Print and shaded views of the part. All mm, measured from the part's lowest x, y and z. A direction names the side the tool comes from. Round coordinates to 2 decimals unless told otherwise and drop trailing zeros. Loops run counter-clockwise (first coordinate to the right, second up) from the corner with the lowest first, then second, coordinate; pieces in that order, holes last. Notation, with made-up numbers: M 34,24.5 L 63,24.5 A9 ccw 63,30.5 Z; hole C -24.75,12.5 d9. An arc over 180 degrees is marked long. One line per item, written item: value. Start each with the question number.
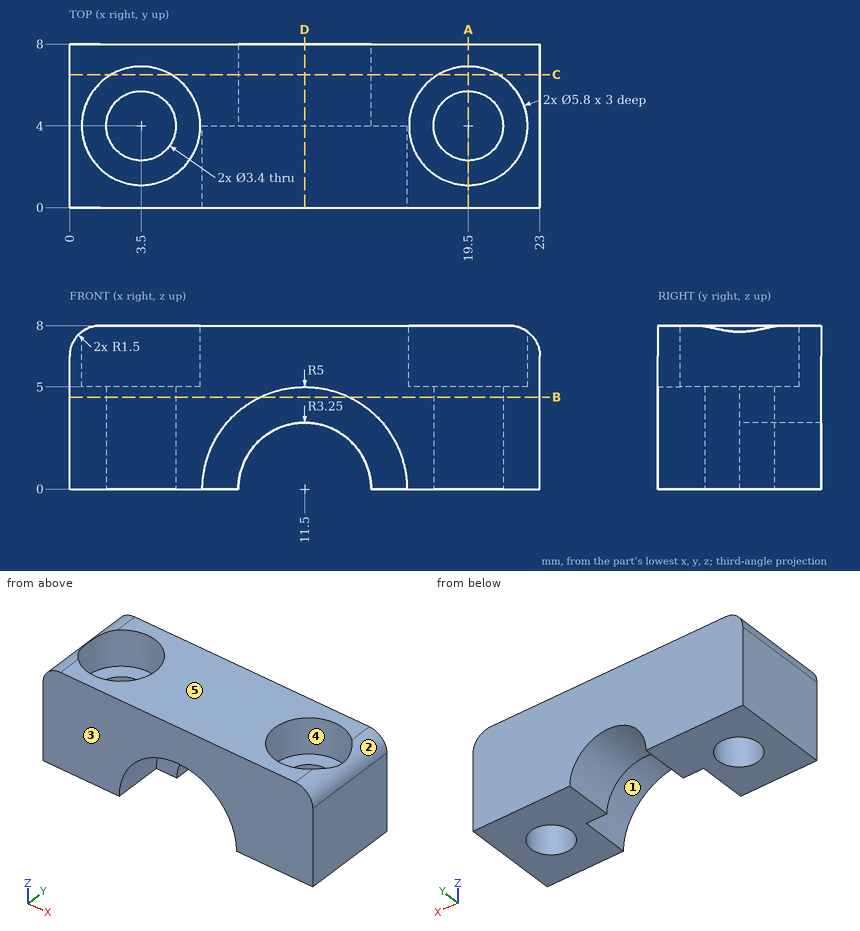
(1) Probe L1, parallel to Y at x = 3.5, z = 2.05; L2, parallel to Y at x = 3.5, z = 7.45; L3, parallel to X at y = 2.5, z = 0.75. List the from-to ranges inside material, lowest first.
(2) Slice it at D-D, the plane x = 11.5. List the corners of the cut face in (y, z), and give its area (3 significant figures).
(3) Flat gauge pins, fed straight in: P1, Ø2, axis at x = 3.5, y = 4, coming from the -Z side; P2, Ø3, axis at x = 4, y = 5, coming from the +Z side; P3, Ø2, axis at x = 11, y = 4.5, coming from the -Z side. Where does each tip first touch, or does it go through?
(4) Slice it at C-C, the plane y = 6.5. List the corners of the cut face in (x, z).
(5) Which spindle directions (+Z, -Z, +X, -X, +Y, -Y) get a long thin tool onto all of the face, cutting with end or side? Do the marked faces 4 and 5. Say none if no direction does.
(6) Slice it at A-A, the plane x = 19.5. List the corners of the cut face in (y, z).
(7) Slice it at B-B, the plane z = 4.5. List the corners of the cut face in (x, y), and give its area (3 significant figures).
(8) Mould opens along X. For the marked faces 1, 2 and 3 say: pulls with the +X half, pulls with the -X half, needs draft (parallel to the pull), parting line crosses it, or undercut.
Check result:
1. L1: y = 0 to 2.3, 5.7 to 8
1. L2: y = 0 to 1.1, 6.9 to 8
1. L3: x = 0 to 2.7, 4.3 to 6.56, 16.44 to 18.7, 20.3 to 23
2. outline: M 0,5 L 4,5 L 4,3.25 L 8,3.25 L 8,8 L 0,8 Z
2. area: 31.0 mm^2
3. P1: passes through
3. P2: stops at z = 5
3. P3: stops at z = 2.88
4. outline: M 0,0 L 8.25,0 A3.25 cw 14.75,0 L 23,0 L 23,6.5 A1.5 ccw 21.5,8 L 20.97,8 L 20.97,5 L 18.03,5 L 18.03,8 L 4.97,8 L 4.97,5 L 2.03,5 L 2.03,8 L 1.5,8 A1.5 ccw 0,6.5 Z
5. face 4: +Z
5. face 5: +Z, +X, -X, +Y, -Y
6. outline: M 0,0 L 2.3,0 L 2.3,5 L 1.1,5 L 1.1,8 L 0,8 Z; M 5.7,0 L 8,0 L 8,8 L 6.9,8 L 6.9,5 L 5.7,5 Z
7. outline: M 0,0 L 9.32,0 L 9.32,4 L 13.68,4 L 13.68,0 L 23,0 L 23,8 L 0,8 Z; hole C 3.5,4 d3.4; hole C 19.5,4 d3.4
7. area: 148 mm^2
8. face 1: undercut
8. face 2: pulls with the +X half
8. face 3: needs draft
